For this review, take the finished solid that the model builds, in its own axes (mm). Give positions to 0.01 mm unless a question says otherwise; leave off trailing zeros. Write each loop counter-clockwise with the first axis right and the second up, starting at its lowest first coordinate (ties: lowest second). Pieces come first, ordered by that corner, then holes. Notation, with made-up numbers: (20.5, -0.5) -> (72.5, -0.5) arc R21 cw to (72.5, 14.5) -> close; hole circle Ø7 at (78.25, -2.5). An arc over 180 degrees is marked (long way). Answer as CSV lines item,"result".
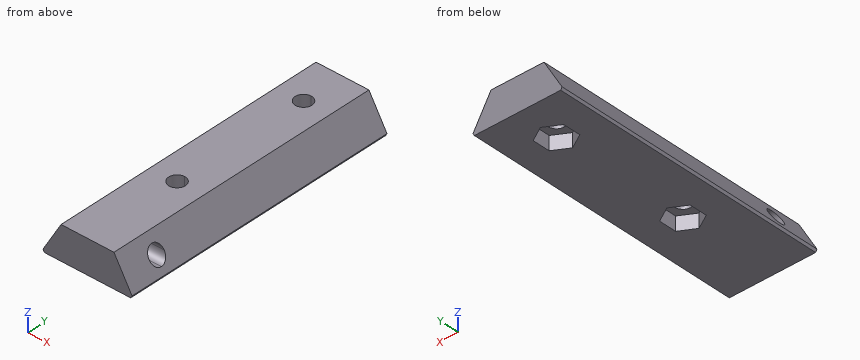
```python
from build123d import *

# Parameters (mm, degrees)
F1_DEPTH      = 50.4
F3_DEPTH      = 6.001
F4_DEPTH      = 2.5
F6_DEPTH      = 8.251
F6_DEPTH_BACK = 8.251
F7_SIZE       = 0.5


with BuildPart() as f1:
    # F0 (on Front) → F1 (new body)
    with BuildSketch(Plane.XZ):
        Polygon((8.25, 0), (4.75, 6), (-4.75, 6), (-8.25, 0), align=None)
    extrude(amount=F1_DEPTH)

    # F2 (on Top) → F3 (cut, through all)
    with BuildSketch(Plane.XY):
        with BuildLine():
            ThreePointArc((1.5, -32.7), (1.0606601718, -31.6393398282), (0, -31.2))
            ThreePointArc((0, -31.2), (-1.0606601718, -33.7606601718), (1.5, -32.7))
        make_face()
        with BuildLine():
            ThreePointArc((0, -6.2), (-1.5, -7.7), (0, -9.2))
            Line((0, -9.2), (0, -6.2))
        make_face()
        with BuildLine():
            Line((0, -6.2), (0, -9.2))
            ThreePointArc((0, -9.2), (1.0606601718, -8.7606601718), (1.5, -7.7))
            ThreePointArc((1.5, -7.7), (1.0606601718, -6.6393398282), (0, -6.2))
        make_face()
    extrude(amount=F3_DEPTH, mode=Mode.SUBTRACT)

    # F2 (on Top) → F4 (cut)
    with BuildSketch(Plane.XY):
        Polygon((2.75, -31.1122867597), (0, -29.5245735195), (-2.75, -31.1122867597), (-2.75, -34.2877132403), (0, -35.8754264805), (2.75, -34.2877132403), align=None)
        with BuildLine():
            ThreePointArc((1.5, -32.7), (-1.0606601718, -33.7606601718), (0, -31.2))
            ThreePointArc((0, -31.2), (1.0606601718, -31.6393398282), (1.5, -32.7))
        make_face(mode=Mode.SUBTRACT)
        with BuildLine():
            Line((-2.75, -9.2877132403), (0, -10.8754264805))
            Line((0, -10.8754264805), (0, -9.2))
            ThreePointArc((0, -9.2), (-1.5, -7.7), (0, -6.2))
            Line((0, -6.2), (0, -4.5245735195))
            Line((0, -4.5245735195), (-2.75, -6.1122867597))
            Line((-2.75, -6.1122867597), (-2.75, -9.2877132403))
        make_face()
        with BuildLine():
            Line((0, -9.2), (0, -10.8754264805))
            Line((0, -10.8754264805), (2.75, -9.2877132403))
            Line((2.75, -9.2877132403), (2.75, -6.1122867597))
            Line((2.75, -6.1122867597), (0, -4.5245735195))
            Line((0, -4.5245735195), (0, -6.2))
            ThreePointArc((0, -6.2), (1.0606601718, -6.6393398282), (1.5, -7.7))
            ThreePointArc((1.5, -7.7), (1.0606601718, -8.7606601718), (0, -9.2))
        make_face()
    extrude(amount=F4_DEPTH, mode=Mode.SUBTRACT)

    # F5 (on Right) → F6 (cut, two sides)
    with BuildSketch(Plane.YZ) as f6_sk:
        with BuildLine():
            ThreePointArc((-43.9, 4.5), (-45.4, 3), (-43.9, 1.5))
            Line((-43.9, 1.5), (-43.9, 4.5))
        make_face()
        with BuildLine():
            Line((-43.9, 4.5), (-43.9, 1.5))
            ThreePointArc((-43.9, 1.5), (-42.8393398282, 1.9393398282), (-42.4, 3))
            ThreePointArc((-42.4, 3), (-42.8393398282, 4.0606601718), (-43.9, 4.5))
        make_face()
    extrude(amount=-F6_DEPTH, mode=Mode.SUBTRACT)
    extrude(f6_sk.sketch, amount=F6_DEPTH_BACK, mode=Mode.SUBTRACT)

    # F7
    f7_edges = [f1.edges().sort_by_distance(p)[0] for p in [
        (-8.25, -25.2, 0),
        (8.25, -25.2, 0),
    ]]
    chamfer(f7_edges, length=F7_SIZE)


solid = f1.part
```
Q1. Add section A-A (x = 3.5). Write out the cut boundary in (y, z).
Answer block:
outline,"(-50.4, 0) -> (0, 0) -> (0, 6) -> (-50.4, 6) -> close; hole circle Ø3 at (-43.9, 3)"
Q2. To check wall thickness, follow probe 1 along Y at (x, z) = (1.25, 1.25); probe 2 along Y at (x, z) = (-0.25, 5.25); probe 3 along Y at (x, z) = (-3.25, 3). State the ranges of each line that lie inside material, in increasing order. Write a range as [from, to].
Answer block:
probe 1,"y = [-50.4, -35.15], [-30.25, -10.15], [-5.25, 0]"
probe 2,"y = [-50.4, -34.18], [-31.22, -9.18], [-6.22, 0]"
probe 3,"y = [-50.4, -45.4], [-42.4, 0]"
Q3. Clearance check with flat-ended pins moving along their axes: pin 1 (2 mm diameter, centred on y = -32, z = 2, fed in from -X); pin 2 (2 mm diameter, centred on y = -45, z = 2, fed in from +X); pin 3 (1.5 mm diameter, centred on y = -7.5, z = 4.5, fed in from +X); pin 4 (2.5 mm diameter, centred on x = 0, y = -32.7, fed in from -Z). State where each tip first meets the part, or that it passes through.
Answer block:
pin 1,"stops at x = -7.67"
pin 2,"stops at x = 7.67"
pin 3,"stops at x = 6.06"
pin 4,"passes through"
Q4. Add section C-C (y = -18). Write out the cut boundary in (x, z), plus the area to 3 significant figures.
Answer block:
outline,"(-8, 0.43) -> (-7.75, 0) -> (7.75, 0) -> (8, 0.43) -> (4.75, 6) -> (-4.75, 6) -> close"
area,"77.8 mm2"
Q5. Add section B-B (z = 3.5). Write out the cut boundary in (x, y), plus the area to 3 significant figures.
Answer block:
outline,"(-6.21, -50.4) -> (6.21, -50.4) -> (6.21, -45.31) -> (-6.21, -45.31) -> close; (-6.21, -42.49) -> (6.21, -42.49) -> (6.21, 0) -> (-6.21, 0) -> close; hole circle Ø3 at (0, -32.7); hole circle Ø3 at (0, -7.7)"
area,"577 mm2"
